Source: three-view drawing plus pictorial views. Frame: mm from the lowest corner of the part. Give positions to 0.01 mm unless a question says otherwise; leave off trailing zeros. Write each loop counter-clockwise with the first axis right and the second up, starting at its lowest first coordinate (ties: lowest second). Pieces come first, ordered by that corner, then holes. Notation, with made-up numbers: (81, 70) -> (135, 70) arc R34 ccw to (135, 103) -> close; hole circle Ø4 at (7, 44). An arc over 180 degrees is marked (long way). Answer in a Markdown table with one row per item. Add a question column.
Item 1: Section query C-C on z = 31.5. Output: boundary loops of the cut face in (x, y).
Item 2: Material intervals for probe 1 along Y at (x, z) = (0.75, 26); probe 2 along Y at (x, z) = (0.6, 25.5) (1 decimal); probe 3 along Z at (x, y) = (0.9, 19), sorted ascending. Write a range as from..to.
Item 3: First-contact query: P1, Ø2, axis at y = 14.75, z = 45.49, coming from the -X side; P2, Ø1, axis at x = 1, y = 27.5, coming from the +Z side. Flat tips, straight axial feed; report the tip coordinate or a pass-through.
Item 4: Section query D-D on x = 1. State how many separate pieces and enclosed holes the cut face has, plus the area to 3 significant figures.
Item 5: Section query B-B on y = 26. Output: boundary loops of the cut face in (x, z).
Item 6: Section query A-A on z = 26. Output: boundary loops of the cut face in (x, y).
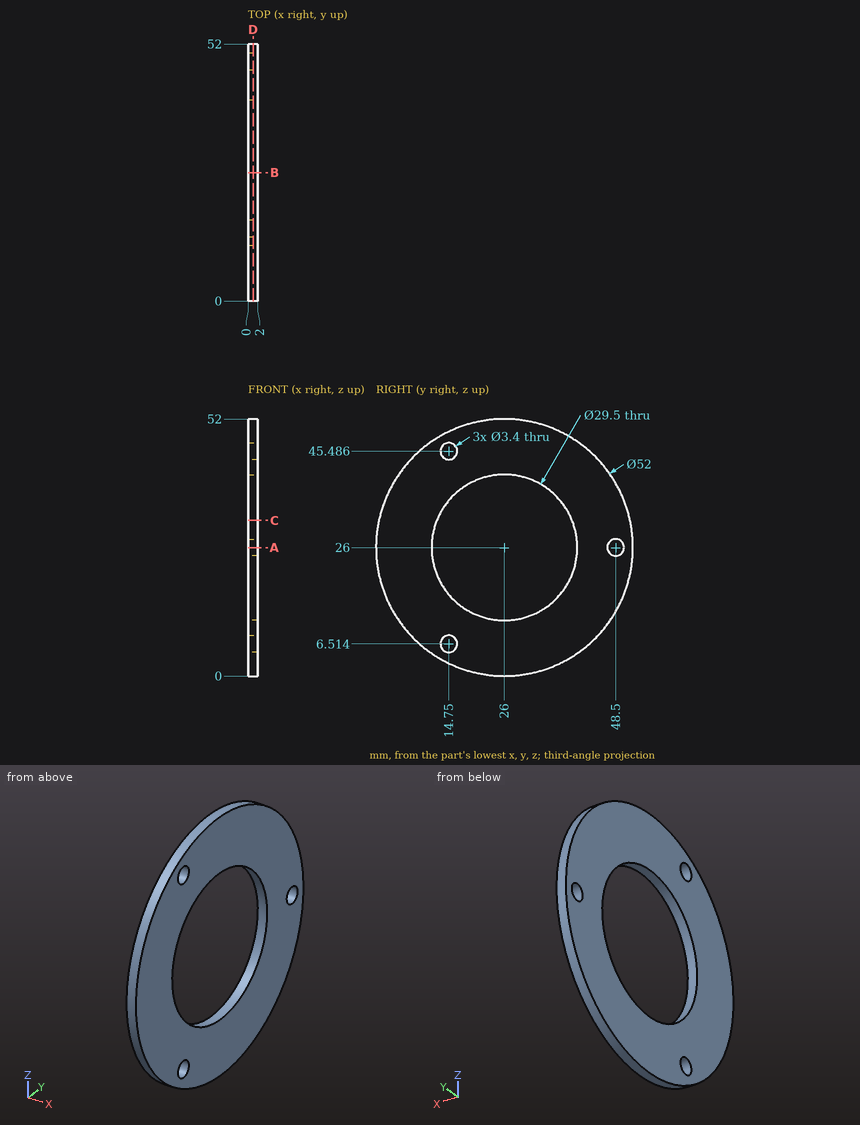
Findings below:
| question | item | result |
|---|---|---|
| 1 | outline | (0, 0.59) -> (2, 0.59) -> (2, 12.31) -> (0, 12.31) -> close; (0, 39.69) -> (2, 39.69) -> (2, 51.41) -> (0, 51.41) -> close |
| 2 | probe 1 | y = 0..11.25, 40.75..46.8, 50.2..52 |
| 2 | probe 2 | y = 0..11.3, 40.7..46.9, 50.1..52 |
| 2 | probe 3 | z = 0.96..13.02, 38.98..51.04 |
| 3 | P1 | passes through |
| 3 | P2 | stops at z = 51.98 |
| 4 | separate pieces | 1 |
| 4 | enclosed holes | 4 |
| 4 | area | 1,410 mm^2 |
| 5 | outline | (0, 0) -> (2, 0) -> (2, 11.25) -> (0, 11.25) -> close; (0, 40.75) -> (2, 40.75) -> (2, 52) -> (0, 52) -> close |
| 6 | outline | (0, 0) -> (2, 0) -> (2, 11.25) -> (0, 11.25) -> close; (0, 40.75) -> (2, 40.75) -> (2, 46.8) -> (0, 46.8) -> close; (0, 50.2) -> (2, 50.2) -> (2, 52) -> (0, 52) -> close |
